Design review of the part built by this model. Coordinates are the model's own, in mm. Round coordinates to 2 decimals unless told otherwise and drop trailing zeros. Write each loop counter-clockwise with the first axis right and the second up, starting at its lowest first coordinate (ties: lowest second). Pieces come first, ordered by that corner, then holes. Notation, with made-up numbers: (47.25, -15.5) -> (66.25, -15.5) arc R25 cw to (66.25, -0.5) -> close; hole circle Ø6 at (28.25, 1.5). An arc over 180 degrees is marked (long way). Write item = value, one per line. Start each with the question number.
Item 1: Add section B-B, the plane y = 5. State the section outline as (x, z) points.
Item 2: Add section D-D, the plane x = -4.5. State the section outline as (y, z) points, then the cut area to 3 significant figures.
Item 3: For pin 1 Ø2 at (x, z) = (-4.5, -10) entering from -Y; pin 2 Ø1 at (y, z) = (6, -16.5) entering from -X, all flat-tipped, find the tip position at first contact; note any pin that passes through.
Item 4: To check wall thickness, follow L1, parallel to Y at x = -3.35, z = -3; L2, parallel to Z at x = -5.05, y = 6.25; L3, parallel to Z at x = -5.4, y = 6. State the ranges of each line that lie inside material, in increasing order.
Item 5: Add section C-C, the plane z = -17. State the section outline as (x, y) points.
Item 6: Add section A-A, the plane x = -3.2. State the section outline as (y, z) points, then the cut area to 3 significant figures.
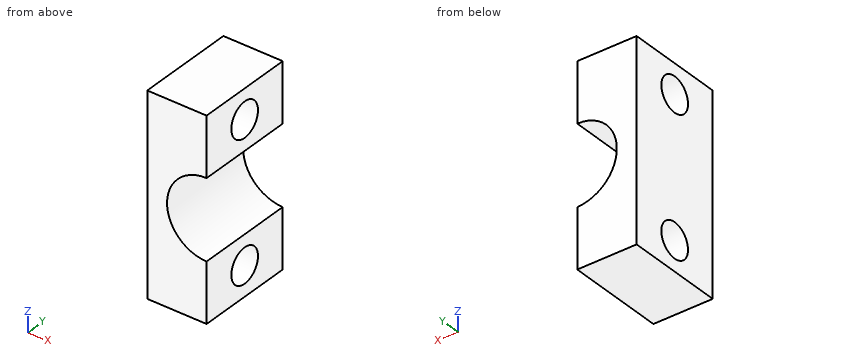
Autodesk Inventor part; units mm, degrees
ref_plane "YZ Plane" through (0, 0, 0) normal (1, 0, 0) x (0, 1, 0)
ref_plane "XZ Plane" through (0, 0, 0) normal (0, 1, 0) x (-1, 0, 0)
ref_plane "XY Plane" through (0, 0, 0) normal (0, 0, 1) x (1, 0, 0)
sketch "Sketch1" plane through (0, 0, 0) normal (0, 1, 0) x (-1, 0, 0)
  line L0 (0, 0) -> (6, 0)
  line L1 (6, 0) -> (6, -20)
  line L2 (6, -20) -> (0, -20)
  arc A0 (0, -14) -> (0, -6) centre (0, -10) ccw
  line L3 (0, -20) -> (0, -14)
  line L4 (0, -6) -> (0, 0)
  dimension "d0" = 6
  dimension "d1" = 20
  dimension "d2" = 6
  dimension "d3" = 20
  dimension "d8" = 8
  dimension "d11" = 90
  dimension "d14" = 6
  dimension "d15" = 6
extrude "Extrusion1" add sketch "Sketch1" along normal blind 10
sketch "Sketch2" plane through (0, 0, 0) normal (1, 0, 0) x (0, 0, -1)
  line L0 (20, 0) -> (14, 0)
  line L1 (20, 0) -> (20, 10)
  line L2 (14, 10) -> (20, 10)
  line L3 (14, 0) -> (14, 10)
  line L4 (6, 0) -> (0, 0)
  line L5 (6, 0) -> (6, 10)
  line L6 (0, 10) -> (6, 10)
  line L7 (0, 0) -> (0, 10)
  circle A0 centre (17, 5) radius 1.75
  circle A1 centre (3, 5) radius 1.75
  dimension "d17" = 3.5
  dimension "d18" = 3.5
  dimension "d20" = 14
  dimension "d21" = 5
  dimension "d22" = 3
  dimension "d23" = 5
extrude "Extrusion2" cut sketch "Sketch2" against normal through all contours A0 | A1
properties part number "reverse gear connecting rod 1"
Result set:
q1.outline = (-6, -20) -> (0, -20) -> (0, -18.75) -> (-6, -18.75) -> close; (-6, -15.25) -> (0, -15.25) -> (0, -14) arc R4 cw to (0, -6) -> (0, -4.75) -> (-6, -4.75) -> close; (-6, -1.25) -> (0, -1.25) -> (0, 0) -> (-6, 0) -> close
q2.outline = (0, -20) -> (10, -20) -> (10, 0) -> (0, 0) -> close; hole circle Ø3.5 at (5, -17); hole circle Ø3.5 at (5, -3)
q2.area = 181 mm²
q3.pin_1 = 0
q3.pin_2 = through
q4.L1 = 0 to 3.25, 6.75 to 10
q4.L2 = -20 to -18.22, -15.78 to -4.22, -1.78 to 0
q4.L3 = -20 to -18.44, -15.56 to -4.44, -1.56 to 0
q5.outline = (-6, 0) -> (0, 0) -> (0, 3.25) -> (-6, 3.25) -> close; (-6, 6.75) -> (0, 6.75) -> (0, 10) -> (-6, 10) -> close
q6.outline = (0, -20) -> (10, -20) -> (10, -12.4) -> (0, -12.4) -> close; (0, -7.6) -> (10, -7.6) -> (10, 0) -> (0, 0) -> close; hole circle Ø3.5 at (5, -17); hole circle Ø3.5 at (5, -3)
q6.area = 133 mm²
